CAD build for the part. Positions are in the model's coordinates, mm. Coordinates: 2 decimals unless noted, no trailing zeros. Order: outer loops, then holes, each group sorted by start corner. A loop starts at its lowest first (then second) coordinate and runs counter-clockwise, first axis right, second up. Notation, with made-up numbers: (38.5, 78) - (97.5, 78) arc R15 cw to (97.5, 96) - close; hole circle Ø10 at (85, 76). An arc over 180 degrees is marked (long way). Use one line per item in the form item = value.
```python
from build123d import *

# Parameters (mm, degrees)
SKETCH1_W           = 11
SKETCH1_H           = 180
BOSS_EXTRUDE1_DEPTH = 1.5
CHAMFER1_SIZE       = 1.5
CHAMFER2_SIZE       = 1.5


with BuildPart() as part:
    # Sketch1 → Boss-Extrude1 (new, symmetric)
    with BuildSketch(Plane.XY):
        Polygon((90, -80), (0, 0), (0, 180), (90, 0), align=None)
        with Locations((-5.5, 90)):
            Rectangle(SKETCH1_W, SKETCH1_H)
    extrude(amount=BOSS_EXTRUDE1_DEPTH, both=True)

    # Chamfer1
    chamfer1_edges = [part.edges().sort_by_distance(p)[0] for p in [
        (45, 90, -1.5),
        (45, 90, 1.5),
    ]]
    chamfer(chamfer1_edges, length=CHAMFER1_SIZE - 0.0001)  # a hair under: the kernel refuses the full size

    # Chamfer2
    chamfer2_edges = [part.edges().sort_by_distance(p)[0] for p in [
        (45, -40, 1.5),
        (45, -40, -1.5),
    ]]
    chamfer(chamfer2_edges, length=CHAMFER2_SIZE - 0.0001)  # a hair under: the kernel refuses the full size


solid = part.part
```
Item 1: Drop a flat-ended pin along its axis: pin 1 (1 mm diameter, centred on y = 121.5, z = 0.5, fed in from +X). Give the stop position or say it passes through.
Derived:
pin_1 = 29.3
Item 2: Cut at C-C, the plane z = 0.8. Write the cut outline in (x, y).
Derived:
outline = (-11, 0) - (1.2, 0) - (90, -78.93) - (90, -1.79) - (-0.89, 180) - (-11, 180) - close
Item 3: Drill centre lines: line 1 (Y direction, x = 45.5, z = 0.15); line 2 (X direction, y = 160.5, z = -0.45); line 3 (X direction, y = -67, z = 0.75). Where is each one in solid material? Low to high. Write a range as [from, to].
Derived:
line_1 = [-40.24, 88.66]
line_2 = [-11, 9.25]
line_3 = [76.5, 90]
